```python
from build123d import *

# Parameters (mm, degrees)
SKETCH1_W                                         = 114.3
SKETCH1_H                                         = 101.6
BOSS_EXTRUDE1_DEPTH                               = 12.7
CBORE_FOR_5_16_SOCKET_HEAD_CAP_SCREW1_D           = 8.4328
CBORE_FOR_5_16_SOCKET_HEAD_CAP_SCREW1_CBORE_D     = 13.49502
CBORE_FOR_5_16_SOCKET_HEAD_CAP_SCREW1_CBORE_DEPTH = 7.9375
M5_CLEARANCE_HOLE1_D                              = 5.5


with BuildPart() as part:
    # Sketch1 → Boss-Extrude1 (new body)
    with BuildSketch(Plane(origin=(0, 0, 0), x_dir=(1, 0, 0), z_dir=(0, 1, 0))):
        with Locations((57.15, 50.8)):
            Rectangle(SKETCH1_W, SKETCH1_H)
    extrude(amount=BOSS_EXTRUDE1_DEPTH)

    # CBORE for 5/16 Socket Head Cap Screw1 (through all)
    with Locations(Plane(origin=(0, 12.7, 0), x_dir=(1, 0, 0), z_dir=(0, 1, 0))):
        with Locations((38.1, 69.85), (76.2, 69.85), (76.2, 31.75), (38.1, 31.75)):
            CounterBoreHole(CBORE_FOR_5_16_SOCKET_HEAD_CAP_SCREW1_D / 2, CBORE_FOR_5_16_SOCKET_HEAD_CAP_SCREW1_CBORE_D / 2, CBORE_FOR_5_16_SOCKET_HEAD_CAP_SCREW1_CBORE_DEPTH)

    # M5 Clearance Hole1 (through all)
    with Locations(Plane(origin=(0, 12.7, 0), x_dir=(1, 0, 0), z_dir=(0, 1, 0))):
        with Locations((17.4625, 11.1125), (96.8375, 11.1125), (96.8375, 90.4875), (17.4625, 90.4875)):
            Hole(M5_CLEARANCE_HOLE1_D / 2)


solid = part.part
```
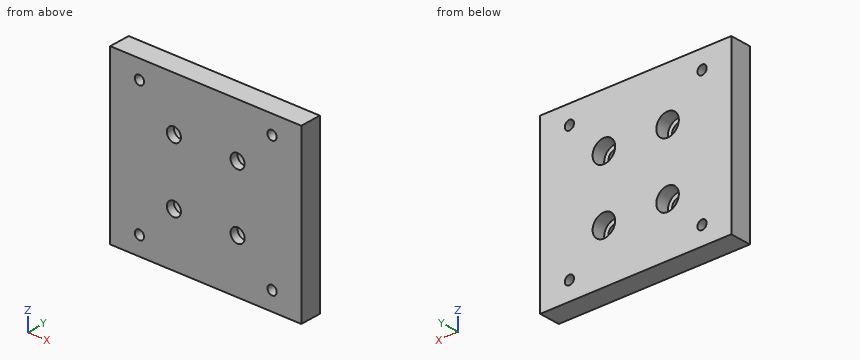
Verification items for the finished model (mm, model axes). Round coordinates to 2 decimals unless told otherwise and drop trailing zeros. Write each loop counter-clockwise with the first axis right and the second up, starting at its lowest first coordinate (ties: lowest second). Pieces come first, ordered by that corner, then holes.
1. Section check C-C on y = 10.5. State how many separate pieces and enclosed holes the cut face has, plus the area to 3 significant figures.
2. Section check A-A on z = -31.75. Enter the section's corners in (x, y).
3. Gauge pin test, flat ends, axial feed: P1, Ø5, axis at x = 17.46, z = -11.11, coming from the -Y side; P2, Ø15.5, axis at x = 76.2, z = -31.75, coming from the -Y side; P3, Ø6.5, axis at x = 79.5, z = -31, coming from the +Y side. Record the tip position at first contact, or that the pin passes through.
4. Scan lines: L1, parallel to Z at x = 38.1, y = 3.45; L2, parallel to Z at x = 38.1, y = 10.5; L3, parallel to X at y = 2.1, z = -31.75. Record each from-to range of solid material in increasing order.
5. Section check B-B on x = 76.2. Enter the section's corners in (y, z), plus the area to 3 significant figures.
6. Section check D-D on x = 18. Enter the section's corners in (y, z).
Answer:
1. separate pieces: 1
1. enclosed holes: 8
1. area: 10,900 mm2
2. outline: (0, 0) - (33.88, 0) - (33.88, 4.76) - (31.35, 4.76) - (31.35, 12.7) - (0, 12.7) - close; (42.32, 0) - (71.98, 0) - (71.98, 4.76) - (69.45, 4.76) - (69.45, 12.7) - (44.85, 12.7) - (44.85, 4.76) - (42.32, 4.76) - close; (80.42, 0) - (114.3, 0) - (114.3, 12.7) - (82.95, 12.7) - (82.95, 4.76) - (80.42, 4.76) - close
3. P1: passes through
3. P2: stops at y = 0
3. P3: stops at y = 4.76
4. L1: z = -101.6 to -74.07, -65.63 to -35.97, -27.53 to 0
4. L2: z = -101.6 to -76.6, -63.1 to -38.5, -25 to 0
4. L3: x = 0 to 33.88, 42.32 to 71.98, 80.42 to 114.3
5. outline: (0, -101.6) - (12.7, -101.6) - (12.7, -76.6) - (4.76, -76.6) - (4.76, -74.07) - (0, -74.07) - close; (0, -65.63) - (4.76, -65.63) - (4.76, -63.1) - (12.7, -63.1) - (12.7, -38.5) - (4.76, -38.5) - (4.76, -35.97) - (0, -35.97) - close; (0, -27.53) - (4.76, -27.53) - (4.76, -25) - (12.7, -25) - (12.7, 0) - (0, 0) - close
5. area: 996 mm2
6. outline: (0, -101.6) - (12.7, -101.6) - (12.7, -93.18) - (0, -93.18) - close; (0, -87.79) - (12.7, -87.79) - (12.7, -13.81) - (0, -13.81) - close; (0, -8.42) - (12.7, -8.42) - (12.7, 0) - (0, 0) - close
